Source: CAD feature listing. Evaluate the final solid. Frame: model axes, mm. A direction names the side the tool comes from. Give positions to 0.01 mm unless a question says otherwise; leave off trailing zeros. Order: outer loops, then holes, each group sorted by start corner. A loop starts at its lowest first (then second) coordinate and runs counter-clockwise, first axis right, second up.
from build123d import *

# Parameters (mm, degrees)
F0_W     = 60
F0_H     = 60
F1_DEPTH = 18.5
F2_R     = 17.5
F4_DEPTH = 17.5
F3_R     = 17.4998645961
F5_DEPTH = 17.5


with BuildPart() as f1:
    # F0 (on Front) → F1 (new body, symmetric)
    with BuildSketch(Plane.XZ):
        Rectangle(F0_W, F0_H)
    extrude(amount=F1_DEPTH, both=True)

    # F2 (on face) → F4 (join)
    with BuildSketch(Plane.XZ.offset(18.5)):
        Circle(F2_R)
    extrude(amount=F4_DEPTH)

    # F3 (on face) → F5 (join)
    with BuildSketch(Plane(origin=(0, 18.5, 0), x_dir=(-1, 0, 0), z_dir=(0, 1, 0))):
        Circle(F3_R)
    extrude(amount=F5_DEPTH)


solid = f1.part
1) First-contact query: pin 1 Ø5 at (y, z) = (28.5, -8.5) entering from +X; pin 2 Ø10 at (y, z) = (24, -13.5) entering from +X; pin 3 Ø6 at (x, z) = (8.5, 21) entering from -Y; pin 4 Ø1.5 at (x, z) = (-2.5, -18) entering from +Y. Flat tips, straight axial feed; report the tip coordinate or a pass-through.
Checks:
pin 1: stops at x = 16.44
pin 2: stops at x = 15.3
pin 3: stops at y = -18.5
pin 4: stops at y = 36
2) Section query A-A on z = 0. Output: boundary loops of the cut face in (x, y), and give its area (4 significant figures).
Checks:
outline: (-30, -18.5) - (-17.5, -18.5) - (-17.5, -36) - (17.5, -36) - (17.5, -18.5) - (30, -18.5) - (30, 18.5) - (17.5, 18.5) - (17.5, 36) - (-17.5, 36) - (-17.5, 18.5) - (-30, 18.5) - close
area: 3,445 mm2
3) Section query D-D on x = 26. Output: boundary loops of the cut face in (y, z), and give its area (3 significant figures).
Checks:
outline: (-18.5, -30) - (18.5, -30) - (18.5, 30) - (-18.5, 30) - close
area: 2,220 mm2
4) Section query C-C on y = -27. Output: boundary loops of the cut face in (x, z), and give its area (3 significant figures).
Checks:
outline: circle Ø35 at (0, 0)
area: 962 mm2
5) Reachability of faces 1 (the face through (0, -36, 0)), 2 (the face through (-14, -18.5, 14)), 3 (the face through (-14, 18.5, 14)) from +Z, -Z, +X, -X, +Y, -Y: full face, straight path, thin tool, end or side. Return the list, or none.
Checks:
face 1: +Z, -Z, +X, -X, -Y
face 2: -Y
face 3: +Y
6) Section query B-B on x = 0. Output: boundary loops of the cut face in (y, z), and give its area (4 significant figures).
Checks:
outline: (-36, -17.5) - (-18.5, -17.5) - (-18.5, -30) - (18.5, -30) - (18.5, -17.5) - (36, -17.5) - (36, 17.5) - (18.5, 17.5) - (18.5, 30) - (-18.5, 30) - (-18.5, 17.5) - (-36, 17.5) - close
area: 3,445 mm2
7) Ray query, L1, parallel to Y at x = 1.5, z = 27; L2, parallel to X at y = 23.5, z = -6.5; L3, parallel to Z at x = -5.5, y = 21.5. Return the intervals inside material, ascending.
Checks:
L1: y = -18.5 to 18.5
L2: x = -16.25 to 16.25
L3: z = -16.61 to 16.61
